Part model, mm, in its own coordinate system. Face numbers are marked on the shaded views. A direction names the side the tool comes from. Round coordinates to 2 decimals unless told otherwise and drop trailing zeros. Loops run counter-clockwise (first coordinate to the right, second up) from the corner with the lowest first, then second, coordinate; pieces in that order, holes last.
1) Mould opens along X. For the marked faces 4, 5 and 6 say: +X half, -X half, draft (parallel to the pull), parting line (faces both ways), or undercut.
2) Band-saw the part on D-D, the plane y = -1. Write the cut outline in (x, z).
3) Drop flat-ended pins along their axis: P1, Ø4, axis at x = -33.5, y = -14, coming from the +Z side; P2, Ø4.5, axis at x = 43.5, y = -12.5, coming from the +Z side; P3, Ø3.5, axis at x = 52, y = 28.5, coming from the -Z side. Give the stop position or say it passes through.
4) Probe line 1 (Y direction, x = -52, z = 6.25); line 2 (Y direction, x = 43.5, z = 1.6); line 3 (Y direction, x = 26, z = 6.5). List the from-to ranges inside material, lowest first.
5) 3-axis set-ups, long thin cutter, end or side, ignore diameter. For the marked faces 1, 2 and 3: which of +Z, -Z, +X, -X, +Y, -Y reach the whole face in a straight line?
6) Band-saw the part on B-B, the plane y = -8.5. Write the cut outline in (x, z).
7) Band-saw the part on A-A, the plane x = -6.5. Write the cut outline in (y, z).
8) Band-saw the part on C-C, the plane x = -52. Write the cut outline in (y, z).
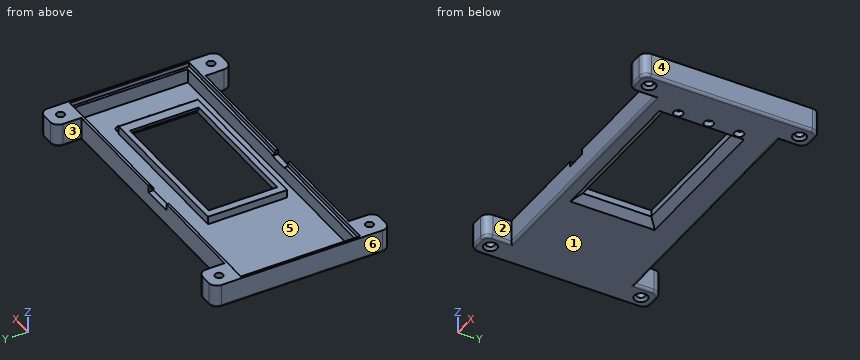
from build123d import *

# Parameters (mm, degrees)
SKETCH_W         = 114
SKETCH_H         = 47
PAD_DEPTH        = 9
THICKNESS_T      = -2
SKETCH004_W      = 10
SKETCH004_H      = 9
PAD001_DEPTH     = 10
SKETCH005_W      = 10
SKETCH005_H      = 9
PAD002_DEPTH     = 10
SKETCH006_W      = 112.2
SKETCH006_H      = 45.2
POCKET_DEPTH     = 1.6
SKETCH007_R      = 1.5
POCKET001_DEPTH  = 9
SKETCH008_W      = 51.5
SKETCH008_H      = 26
POCKET002_DEPTH  = 7
SKETCH009_W      = 58.5
SKETCH009_H      = 30
PAD003_DEPTH     = 3
SKETCH010_W      = 51.5
SKETCH010_H      = 26
POCKET003_DEPTH  = 3
SKETCH011_R      = 1.75
POCKET004_DEPTH  = 2
CHAMFER_SIZE     = 1
CHAMFER001_ANGLE = 45
CHAMFER001_SIZE  = 4
CHAMFER002_ANGLE = 40
CHAMFER002_SIZE  = 3
FILLET_R         = 3
FILLET001_R      = 3
FILLET002_R      = 1
FILLET003_R      = 1
FILLET004_R      = 1
SKETCH012_W      = 12
SKETCH012_H      = 2.5
POCKET005_DEPTH  = 2
SKETCH013_W      = 8
SKETCH013_H      = 2
POCKET006_DEPTH  = 2


with BuildPart() as part:
    # Sketch → Pad (new body)
    with BuildSketch(Plane.XY):
        Rectangle(SKETCH_W, SKETCH_H)
    extrude(amount=PAD_DEPTH)

    # Thickness
    thickness_openings = [part.faces().sort_by_distance(p)[0] for p in [
        (0, 0, 9),
    ]]
    offset(amount=THICKNESS_T, openings=thickness_openings)

    # Sketch004 → Pad001 (join)
    with BuildSketch(Plane.XZ.offset(23.5)):
        with Locations((-52, 4.5)):
            Rectangle(SKETCH004_W, SKETCH004_H)
        with Locations((52, 4.5)):
            Rectangle(SKETCH004_W, SKETCH004_H)
    extrude(amount=PAD001_DEPTH)

    # Sketch005 (on Face1 of Pad001) → Pad002 (join)
    with BuildSketch(Plane(origin=(0, 23.5, 0), x_dir=(-1, 0, 0), z_dir=(0, 1, 0))):
        with Locations((-52, 4.5)):
            Rectangle(SKETCH005_W, SKETCH005_H)
        with Locations((52, 4.5)):
            Rectangle(SKETCH005_W, SKETCH005_H)
    extrude(amount=PAD002_DEPTH)

    # Sketch006 (on Face12 of Pad002) → Pocket (cut)
    with BuildSketch(Plane.XY.offset(9)):
        Rectangle(SKETCH006_W, SKETCH006_H)
    extrude(amount=-POCKET_DEPTH, mode=Mode.SUBTRACT)

    # Sketch007 (on Face2 of Pocket) → Pocket001 (cut)
    with BuildSketch(Plane(origin=(0, 0, 0), x_dir=(1, 0, 0), z_dir=(0, 0, -1))):
        with Locations((-52, 28.5)):
            Circle(SKETCH007_R)
        with Locations((52, 28.5)):
            Circle(SKETCH007_R)
        with Locations((52, -28.5)):
            Circle(SKETCH007_R)
        with Locations((-52, -28.5)):
            Circle(SKETCH007_R)
    extrude(amount=-POCKET001_DEPTH, mode=Mode.SUBTRACT)

    # Sketch008 (on Face2 of Pocket001) → Pocket002 (cut)
    with BuildSketch(Plane(origin=(0, 0, 0), x_dir=(1, 0, 0), z_dir=(0, 0, -1))):
        with Locations((11.75, 2.5)):
            Rectangle(SKETCH008_W, SKETCH008_H)
    extrude(amount=-POCKET002_DEPTH, mode=Mode.SUBTRACT)

    # Sketch009 (on Face27 of Pocket002) → Pad003 (join)
    with BuildSketch(Plane.XY.offset(2)):
        with Locations((12.25, -2.5)):
            Rectangle(SKETCH009_W, SKETCH009_H)
    extrude(amount=PAD003_DEPTH)

    # Sketch010 (on Face38 of Pad003) → Pocket003 (cut)
    with BuildSketch(Plane.XY.offset(5)):
        with Locations((11.75, -2.5)):
            Rectangle(SKETCH010_W, SKETCH010_H)
    extrude(amount=-POCKET003_DEPTH, mode=Mode.SUBTRACT)

    # Sketch011 (on Face2 of Pocket003) → Pocket004 (cut)
    with BuildSketch(Plane(origin=(0, 0, 0), x_dir=(1, 0, 0), z_dir=(0, 0, -1))):
        with Locations((43.5, -10.5)):
            Circle(SKETCH011_R)
        with Locations((43.5, 1)):
            Circle(SKETCH011_R)
        with Locations((43.5, 12.5)):
            Circle(SKETCH011_R)
    extrude(amount=-POCKET004_DEPTH, mode=Mode.SUBTRACT)

    # Chamfer
    chamfer_edges = [part.edges().sort_by_distance(p)[0] for p in [
        (50.5, 28.5, 0),
        (50.5, -28.5, 0),
        (-53.5, -28.5, 0),
        (-53.5, 28.5, 0),
    ]]
    chamfer(chamfer_edges, length=CHAMFER_SIZE)

    # Chamfer001
    chamfer001_edges = [part.edges().sort_by_distance(p)[0] for p in [
        (37.5, -2.5, 0),
    ]]
    chamfer001_side = part.faces().sort_by_distance((48.177691, 28.5, 0))[0]
    chamfer(chamfer001_edges, length=CHAMFER001_SIZE, angle=CHAMFER001_ANGLE, reference=chamfer001_side)

    # Chamfer002
    chamfer002_edges = [part.edges().sort_by_distance(p)[0] for p in [
        (11.75, -15.5, 0),
        (-14, -2.5, 0),
        (11.75, 10.5, 0),
    ]]
    chamfer002_side = part.faces().sort_by_distance((39.5, 11.822309, 0))[0]
    chamfer(chamfer002_edges, length=CHAMFER002_SIZE, angle=CHAMFER002_ANGLE, reference=chamfer002_side)

    # Fillet
    fillet_edges = [part.edges().sort_by_distance(p)[0] for p in [
        (57, -33.5, 4.5),
        (47, -33.5, 4.5),
        (-47, -33.5, 4.5),
        (-57, -33.5, 4.5),
    ]]
    fillet(fillet_edges, radius=FILLET_R)

    # Fillet001
    fillet001_edges = [part.edges().sort_by_distance(p)[0] for p in [
        (-57, 33.5, 4.5),
        (-47, 33.5, 4.5),
        (47, 33.5, 4.5),
        (57, 33.5, 4.5),
    ]]
    fillet(fillet001_edges, radius=FILLET001_R)

    # Fillet002
    fillet002_edges = [part.edges().sort_by_distance(p)[0] for p in [
        (-47, 27, 0),
        (-47, -27, 0),
        (-57, 0, 0),
    ]]
    fillet(fillet002_edges, radius=FILLET002_R)

    # Fillet003
    fillet003_edges = [part.edges().sort_by_distance(p)[0] for p in [
        (47, 27, 0),
        (57, 0, 0),
        (47, -27, 0),
    ]]
    fillet(fillet003_edges, radius=FILLET003_R)

    # Fillet004
    fillet004_edges = [part.edges().sort_by_distance(p)[0] for p in [
        (0, 23.5, 0),
        (0, -23.5, 0),
    ]]
    fillet(fillet004_edges, radius=FILLET004_R)

    # Sketch012 (on Face33 of Fillet004) → Pocket005 (cut)
    with BuildSketch(Plane(origin=(0, 23.5, 0), x_dir=(-1, 0, 0), z_dir=(0, 1, 0))):
        with Locations((3, 7.75)):
            Rectangle(SKETCH012_W, SKETCH012_H)
    extrude(amount=-POCKET005_DEPTH, mode=Mode.SUBTRACT)

    # Sketch013 (on Face49 of Pocket005) → Pocket006 (cut)
    with BuildSketch(Plane.XZ.offset(23.5)):
        with Locations((-4.5, 8)):
            Rectangle(SKETCH013_W, SKETCH013_H)
    extrude(amount=-POCKET006_DEPTH, mode=Mode.SUBTRACT)


solid = part.part
Reported:
1. face 4: +X half
1. face 5: undercut
1. face 6: -X half
2. outline: (-57, 1) arc R1 ccw to (-56, 0) - (-17, 0) - (-14, 2.52) - (-14, 5) - (-17, 5) - (-17, 2) - (-55, 2) - (-55, 7.4) - (-56.1, 7.4) - (-56.1, 9) - (-57, 9) - close; (37.5, 4) - (41.5, 0) - (41.75, 0) - (41.75, 2) - (41.5, 2) - (41.5, 5) - (37.5, 5) - close; (45.25, 0) - (56, 0) arc R1 ccw to (57, 1) - (57, 9) - (56.1, 9) - (56.1, 7.4) - (55, 7.4) - (55, 2) - (45.25, 2) - close
3. P1: stops at z = 2
3. P2: stops at z = 5
3. P3: stops at z = 0.75
4. line 1: y = -33.5 to -30, -27 to -21.5, 21.5 to 27, 30 to 33.5
4. line 2: y = -23.5 to -14.25, -10.75 to -2.75, 0.75 to 8.75, 12.25 to 23.5
4. line 3: y = -23.5 to -21.5, 21.5 to 23.5
5. face 1: -Z, +X, -X, +Y, -Y
5. face 2: +Z, -Z, -Y
5. face 3: +Z, -Z, +Y
6. outline: (-57, 1) arc R1 ccw to (-56, 0) - (-17, 0) - (-14, 2.52) - (-14, 5) - (-17, 5) - (-17, 2) - (-55, 2) - (-55, 7.4) - (-56.1, 7.4) - (-56.1, 9) - (-57, 9) - close; (37.5, 4) - (41.5, 0) - (56, 0) arc R1 ccw to (57, 1) - (57, 9) - (56.1, 9) - (56.1, 7.4) - (55, 7.4) - (55, 2) - (41.5, 2) - (41.5, 5) - (37.5, 5) - close
7. outline: (-23.5, 1) arc R1 ccw to (-22.5, 0) - (-18.5, 0) - (-15.5, 2.52) - (-15.5, 5) - (-17.5, 5) - (-17.5, 2) - (-21.5, 2) - (-21.5, 7) - (-23.5, 7) - close; (10.5, 2.52) - (13.5, 0) - (22.5, 0) arc R1 ccw to (23.5, 1) - (23.5, 6.5) - (21.5, 6.5) - (21.5, 2) - (12.5, 2) - (12.5, 5) - (10.5, 5) - close
8. outline: (-33.5, 1) arc R1 ccw to (-32.5, 0) - (-31, 0) - (-30, 1) - (-30, 9) - (-33.5, 9) - close; (-27, 1) - (-26, 0) - (26, 0) - (27, 1) - (27, 9) - (22.6, 9) - (22.6, 7.4) - (21.5, 7.4) - (21.5, 2) - (-21.5, 2) - (-21.5, 7.4) - (-22.6, 7.4) - (-22.6, 9) - (-27, 9) - close; (30, 1) - (31, 0) - (32.5, 0) arc R1 ccw to (33.5, 1) - (33.5, 9) - (30, 9) - close
